Autodesk Inventor part; units mm, degrees
ref_plane "YZ Plane" through (0, 0, 0) normal (1, 0, 0) x (0, 1, 0)
ref_plane "XZ Plane" through (0, 0, 0) normal (0, 1, 0) x (-1, 0, 0)
ref_plane "XY Plane" through (0, 0, 0) normal (0, 0, 1) x (1, 0, 0)
sketch "Sketch1" plane through (0, 0, 0) normal (0, 0, 1) x (1, 0, 0)
  line L0 (-10.2, 5.715) -> (10.2, 5.715)
  line L1 (10.2, 5.715) -> (10.2, -5.715)
  line L2 (10.2, -5.715) -> (-10.2, -5.715)
  line L3 (-10.2, -5.715) -> (-10.2, 5.715)
  point P0 (0, 0)
  dimension "d0" = 20.4
  dimension "d1" = 10.2
  dimension "d2" = 11.43
  dimension "d3" = 5.715
extrude "Extrusion1" add sketch "Sketch1" along normal blind 6.35
sketch "Sketch2" plane through (0, 0, 0) normal (0, 0, -1) x (-1, 0, 0)
  line L0 (8.205, 6.54) -> (7.015, 6.54)
  line L1 (7.015, 6.54) -> (7.015, 4.89)
  line L2 (7.015, 4.89) -> (8.205, 4.89)
  line L3 (8.205, 4.89) -> (8.205, 6.54)
  line L4 (10.2, 5.715) -> (-10.2, 5.715)
  line L5 (10.2, -5.715) -> (10.2, 5.715)
  point P0 (0, 0)
  dimension "d6" = 1.65
  dimension "d7" = 0.825
  dimension "d8" = 1.19
  dimension "d9" = 1.995
extrude "Extrusion2" add sketch "Sketch2" against normal blind 1.27
pattern_linear "Rectangular Pattern1" count 7 spacing 2.54 along (1, 0, 0) of "Extrusion2"
mirror "Mirror1" about plane through (0, 0, 0) normal (0, 1, 0) of "Extrusion2", "Rectangular Pattern1"
properties part number "MC_BK276"
Source: CAD feature listing. Evaluate the final solid. Frame: model axes, mm. A direction names the side the tool comes from. Give positions to 0.01 mm unless a question says otherwise; leave off trailing zeros. Write each loop counter-clockwise with the first axis right and the second up, starting at its lowest first coordinate (ties: lowest second). Pieces come first, ordered by that corner, then holes. Notation, with made-up numbers: M 55,67 L 101,67 A30 cw 101,96 Z; hole C -13,37 d5. An arc over 180 degrees is marked long. Return JSON: item names as keys, results as strings. Group by question number.
1) Material intervals for line 1 along Z through (x, y) = (-7.5, 5.75); line 2 along Y through (x, z) = (6, 5) (3 decimals), sorted ascending. Write a range as [from, to].
2) Pin query (flat end, axial travel): P1, Ø0.9, axis at y = 6, z = 1, coming from the -X side; P2, Ø0.9, axis at x = 5, y = -6.5, coming from the +Z side; P3, Ø0.9, axis at y = -6.5, z = 0.5, coming from the -X side (3 decimals); P4, Ø0.7, axis at y = 6.5, z = 0.5, coming from the +X side (3 decimals). Return the tip coordinate at first contact, or that it passes through.
3) Cut plane B-B, the plane z = 4.5. Output: boundary loops of the cut face in (x, y) (3 decimals), plus the area to 3 significant figures.
4) Cut plane A-A, the plane x = 2.25. Output: boundary loops of the cut face in (y, z) (3 decimals), plus the area to 3 significant figures.
5) Set-up query: faces 1 (the face through (-8, 6, 1.27)), 2 (the face through (3.145, -6, 1)), 3 (the face through (0, -6, 1.27)). Return all of +Z, -Z, +X, -X, +Y, -Y with unobstructed straight access to the full face (end or side cutting, diameter ignored); none if empty.
6) Cut plane C-C, the plane x = -8.75. Output: boundary loops of the cut face in (y, z) (3 decimals).
Recorded:
{
 "1": {"line 1": "z = [0, 1.27]", "line 2": "y = [-5.715, 5.715]"},
 "2": {"P1": "stops at x = -10.2", "P2": "stops at z = 1.27", "P3": "stops at x = -8.205", "P4": "stops at x = 8.225"},
 "3": {"outline": "M -10.2,-5.715 L 10.2,-5.715 L 10.2,5.715 L -10.2,5.715 Z", "area": "233 mm²"},
 "4": {"outline": "M -6.54,0 L 6.54,0 L 6.54,1.27 L 5.715,1.27 L 5.715,6.35 L -5.715,6.35 L -5.715,1.27 L -6.54,1.27 Z", "area": "74.7 mm²"},
 "5": {"face 1": "+Z, +X, -X, +Y", "face 2": "+Z, -Z, -Y", "face 3": "+Z, +X, -X, -Y"},
 "6": {"outline": "M -5.715,0 L 5.715,0 L 5.715,6.35 L -5.715,6.35 Z"}
}
